Part model, mm, in its own coordinate system. A direction names the side the tool comes from. Round coordinates to 2 decimals unless told otherwise and drop trailing zeros. Write each loop counter-clockwise with the first axis right and the second up, starting at its lowest first coordinate (ties: lowest second). Pieces come first, ordered by that corner, then holes.
from build123d import *

# Parameters (mm, degrees)
P_IDAT_VYSUNUT_M1_DEPTH  = 4
SKICA2_W                 = 5
SKICA2_H                 = 8
P_IDAT_VYSUNUT_M2_DEPTH  = 20
SKICA3_W                 = 8
SKICA3_H                 = 5
P_IDAT_VYSUNUT_M3_DEPTH  = 32
P_IDAT_VYSUNUT_M4_DEPTH  = 2.5
SKICA5_R                 = 3
ODEBRAT_VYSUNUT_M1_DEPTH = 15
ZAOBLIT1_R               = 5
SKICA6_R                 = 1.2
ODEBRAT_VYSUNUT_M2_DEPTH = 8
ZAOBLIT2_R               = 4
SKICA7_R                 = 0.95
ODEBRAT_VYSUNUT_M3_DEPTH = 13
ODEBRAT_VYSUNUT_M4_DEPTH = 10
SKICA9_W                 = 1.6
SKICA9_H                 = 3.3
ODEBRAT_VYSUNUT_M5_DEPTH = 10


with BuildPart() as part:
    # Skica1 → Přidat vysunutím1 (new, symmetric)
    with BuildSketch(Plane.XY):
        Polygon((0, 0), (17, 0), (17, 23.5), (0, 23.5), (0, 28.5), (22, 28.5), (22, -5), (0, -5), align=None)
    extrude(amount=P_IDAT_VYSUNUT_M1_DEPTH, both=True)

    # Skica2 → Přidat vysunutím2 (add)
    with BuildSketch(Plane(origin=(0, 28.5, 0), x_dir=(1, 0, 0), z_dir=(0, 1, 0))):
        with Locations((19.5, 0)):
            Rectangle(SKICA2_W, SKICA2_H)
    extrude(amount=P_IDAT_VYSUNUT_M2_DEPTH)

    # Skica3 → Přidat vysunutím3 (add)
    with BuildSketch(Plane.ZY.offset(-17)):
        with Locations((0, 46)):
            Rectangle(SKICA3_W, SKICA3_H)
    extrude(amount=P_IDAT_VYSUNUT_M3_DEPTH)

    # Skica4 → Přidat vysunutím4 (add, symmetric)
    with BuildSketch(Plane.XY):
        Polygon((17, 43.5), (7, 43.5), (17, 38.5), align=None)
    extrude(amount=P_IDAT_VYSUNUT_M4_DEPTH, both=True)

    # Skica5 → Odebrat vysunutím1 (cut)
    with BuildSketch(Plane(origin=(0, 48.5, 0), x_dir=(1, 0, 0), z_dir=(0, 1, 0))):
        with Locations(Location((-2, 0, 0), (0, 0, 270))):
            Circle(SKICA5_R)
    extrude(amount=-ODEBRAT_VYSUNUT_M1_DEPTH, mode=Mode.SUBTRACT)

    # Zaoblit1
    zaoblit1_edges = [part.edges().sort_by_distance(p)[0] for p in [
        (22, -5, 0),
        (22, 48.5, 0),
    ]]
    fillet(zaoblit1_edges, radius=ZAOBLIT1_R)

    # Skica6 → Odebrat vysunutím2 (cut)
    with BuildSketch(Plane.ZY):
        with Locations((-6.1415e-05, 25.09368658)):
            Circle(SKICA6_R)
        with Locations((-5.8558e-05, -1.893787552)):
            Circle(SKICA6_R)
    extrude(amount=-ODEBRAT_VYSUNUT_M2_DEPTH, mode=Mode.SUBTRACT)

    # Zaoblit2
    zaoblit2_edges = [part.edges().sort_by_distance(p)[0] for p in [
        (-15, 46, -4),
        (-15, 46, 4),
    ]]
    fillet(zaoblit2_edges, radius=ZAOBLIT2_R - 0.0001)  # a hair under: the kernel refuses the full size

    # Skica7 → Odebrat vysunutím3 (cut)
    with BuildSketch(Plane(origin=(0, 48.5, 0), x_dir=(1, 0, 0), z_dir=(0, 1, 0))):
        with Locations(Location((-10.5, 0, 0), (0, 0, 270))):
            Circle(SKICA7_R)
        with Locations(Location((6.5, 0, 0), (0, 0, 270))):
            Circle(SKICA7_R)
    extrude(amount=-ODEBRAT_VYSUNUT_M3_DEPTH, mode=Mode.SUBTRACT)

    # Skica8 → Odebrat vysunutím4 (cut)
    with BuildSketch(Plane(origin=(0, 0, 0), x_dir=(1, 0, 0), z_dir=(0, 1, 0))):
        with BuildLine():
            Line((12.5, 2.5), (14.5, 2.5))
            ThreePointArc((14.5, 2.5), (17, 0), (14.5, -2.5))
            Line((14.5, -2.5), (12.5, -2.5))
            ThreePointArc((12.5, -2.5), (10, 0), (12.5, 2.5))
        make_face()
    extrude(amount=-ODEBRAT_VYSUNUT_M4_DEPTH, mode=Mode.SUBTRACT)

    # Skica9 → Odebrat vysunutím5 (cut)
    with BuildSketch(Plane.XY.offset(4)):
        with Locations((17.8, 34.35)):
            Rectangle(SKICA9_W, SKICA9_H)
        with Locations((17.8, 10.1)):
            Rectangle(SKICA9_W, SKICA9_H)
    extrude(amount=-ODEBRAT_VYSUNUT_M5_DEPTH, mode=Mode.SUBTRACT)


solid = part.part
Q1. Saw through at A-A, the plane x = -2. Write the cut outline in (y, z), and give its area (3 significant figures).
Q2. Saw through at C-C, the plane x = -8.5. Write the cut outline in (y, z), and give its area (3 significant figures).
Q3. Wall check: line 1 (Y direction, x = 11, z = 2.75); line 2 (Z direction, x = 6.5, y = 47.05); line 3 (X direction, y = 45.75, z = 0). Give the ranges that are in metal, low to high.
Q4. Drop flat-ended pins along their axis: P1, Ø2.5, axis at y = 19.5, z = 2, coming from the -X side; P2, Ø4, axis at x = 9.5, y = 41, coming from the -Z side; P3, Ø2, axis at y = -1.89, z = 0, coming from the -X side; P4, Ø12, axis at x = -3.5, y = 5.5, coming from the +Z side. Give the stop position or say it passes through.
Q5. Saw through at B-B, the plane y = 3. Write the cut outline in (x, z).
Q6. Tool access for faces 1 (the flat face through (6, 0, 0)), 2 (the flat face through (14, -2, 2.5)), 3 (the cylindrical face through (5.66, 45.92, 0.44)), 4 (the flat face through (8, -2, 0)): list every direction of +Z, -Z, +X, -X, +Y, -Y with a clear straight run to the whole face (end or side of a thin tool).
Q7. Two-plate mould, pull along Y, no slides. Class faces 5 (the flat face through (18, 11.75, 0)), 6 (the flat face through (14, 24, 4)): released by +Y, released by -Y, zero draft, split by the parting line, or undercut.
Computed:
1. outline: (43.5, -4) - (48.5, -4) - (48.5, -3) - (43.5, -3) - close; (43.5, 3) - (48.5, 3) - (48.5, 4) - (43.5, 4) - close
1. area: 10.0 mm2
2. outline: (43.5, -4) - (48.5, -4) - (48.5, 4) - (43.5, 4) - close
2. area: 40.0 mm2
3. line 1: y = -5 to 0, 23.5 to 28.5, 43.5 to 48.5
3. line 2: z = -4 to -0.95, 0.95 to 4
3. line 3: x = -15 to -11.45, -9.55 to -5, 1 to 5.55, 7.45 to 21.47
4. P1: stops at x = 17
4. P2: stops at z = -2.5
4. P3: stops at x = 8
4. P4: passes through
5. outline: (17, -4) - (22, -4) - (22, 4) - (17, 4) - close
6. face 1: +Z, -Z, -X
6. face 2: -Y
6. face 3: +Y
6. face 4: -X
7. face 5: undercut
7. face 6: zero draft
